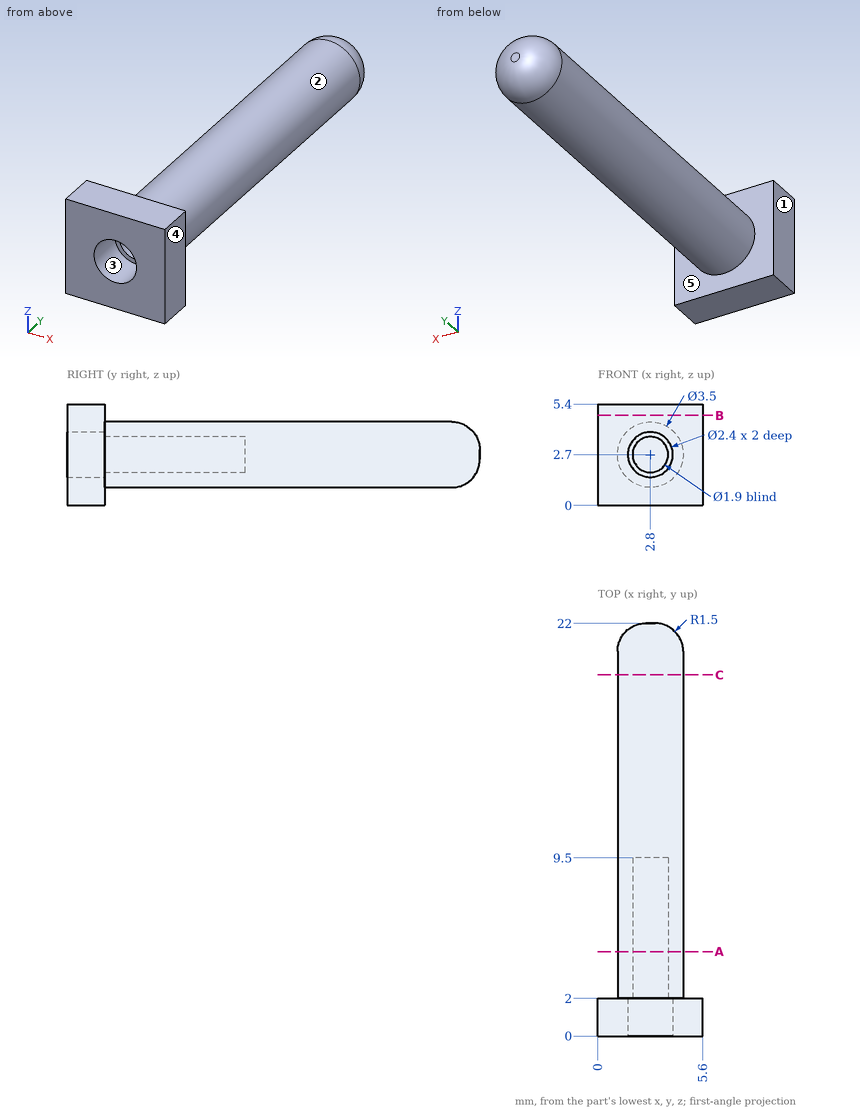
Can you work these out from the drawing? Everything is in mm from the part's minimum corner. A direction names the side the tool comes from. Coordinates: 2 decimals unless noted, no trailing zeros. Order: outer loops, then holes, each group sorted by start corner. A loop starts at its lowest first (then second) coordinate and runs counter-clockwise, first axis right, second up. Notation, with made-up numbers: (-29.75, 1) -> (2.25, 1) arc R14 cw to (2.25, 19) -> close; hole circle Ø5 at (61.25, 41). An arc over 180 degrees is marked (long way). Use one line per item in the form item = value.
Q1. Imagine slicing it at C-C, the plane y = 19.25. List the corners of the cut face in (x, z) for me.
From the geometry:
outline = circle Ø3.5 at (2.8, 2.7)
Q2. I need wall thicknesses on L1, parallel to X at y = 7, z = 2.7; L2, parallel to X at y = 0.7, z = 2.7; L3, parallel to Y at x = 4.6, z = 3.55. Which ranges of each line are inside material? Lowest first, please.
From the geometry:
L1 = 1.05 to 1.85, 3.75 to 4.55
L2 = 0 to 1.6, 4 to 5.6
L3 = 0 to 2
Q3. Imagine slicing it at A-A, the plane y = 4.5. List the corners of the cut face in (x, z) for me.
From the geometry:
outline = circle Ø3.5 at (2.8, 2.7); hole circle Ø1.9 at (2.8, 2.7)
Q4. Which directions (+Z, -Z, +X, -X, +Y, -Y) give clear straight access to the entire face, cutting with the end or side of a thin tool? Please do the marked faces 1 and 2.
From the geometry:
face_1 = +Z, -Z, -X, +Y, -Y
face_2 = +Y
Q5. Imagine slicing it at B-B, the plane z = 4.8. List the corners of the cut face in (x, y) for me.
From the geometry:
outline = (0, 0) -> (5.6, 0) -> (5.6, 2) -> (0, 2) -> close
Q6. Will these pins go through, and if not, where does the flat tip stop? P1, Ø1.1, axis at x = 2.8, z = 2.7, coming from the -Y side; P2, Ø1, axis at x = 4, z = 2.5, coming from the +Y side; P3, Ø1.6, axis at x = 1.5, z = 3, coming from the +Y side.
From the geometry:
P1 = 9.5
P2 = 21.93
P3 = 21.97
Q7. We'd pull the mould along X, two halves only. Please class the marked faces 3, 4 and 5: released by +X, released by -X, zero draft, split by the parting line, or undercut.
From the geometry:
face_3 = undercut
face_4 = released by +X
face_5 = zero draft
